Autodesk Inventor part; units mm, degrees
ref_plane "Work Plane1" through (0, 27, 0) normal (0, 1, 0) x (1, 0, 0)
ref_plane "YZ Plane" through (0, 0, 0) normal (1, 0, 0) x (0, 1, 0)
ref_plane "XZ Plane" through (0, 0, 0) normal (0, 1, 0) x (-1, 0, 0)
sketch "Sketch1" plane through (0, 0, 0) normal (0, 1, 0) x (-1, 0, 0)
  circle A0 centre (0, 0) radius 9.5
  circle A1 centre (0, 0) radius 13
  dimension "d0" = 19
  dimension "d3" = 26
extrude "Extrusion1" add sketch "Sketch1" against normal blind 6.5 contours A0
extrude "Extrusion2" add sketch "Sketch1" along normal blind 2 contours A0 | A1
sketch "Sketch2" plane through (0, 2, 0) normal (0, 1, 0) x (1, 0, 0)
  circle A0 centre (0, 0) radius 13
  circle A1 centre (0, 0) radius 10
  dimension "d6" = 20
ref_plane "Work Plane1" through (0, 27, 0) normal (0, 1, 0) x (1, 0, 0)
sketch "Sketch3" plane through (0, 27, 0) normal (0, 1, 0) x (1, 0, 0)
  circle A0 centre (0, 0) radius 2.5
  dimension "d8" = 5
loft "Loft1" add profiles "Sketch3", "Sketch2" contours all / A1
shell "Shell1" thickness 0.8 removed faces 2 at (1.2612, 27, 0.6619) at (-2.3703, -6.5, -2.0999)
properties part number "Microsuction"
For this review, take the finished solid that the model builds, in its own axes (mm). A direction names the side the tool comes from. Coordinates: 2 decimals unless noted, no trailing zeros. Write each loop counter-clockwise with the first axis right and the second up, starting at its lowest first coordinate (ties: lowest second). Pieces come first, ordered by that corner, then holes. Notation, with made-up numbers: (63, -35.75) - (88, -35.75) arc R11 cw to (88, -25.75) - close; hole circle Ø11 at (61.5, 19). An arc over 180 degrees is marked (long way). Put each result on its own line as item: value.
1. Mouldability with a two-part tool opening along Y and no side actions: class faces 6 (the cylindrical face through (10.316, 0.986, 7.91)), 7 (the flat face through (-8, 0.8, -5)), 8 (the conical face through (-4.34, 17.1, -3.33)) as released by +Y, released by -Y, zero draft, split by the parting line, or undercut.
Values found:
face 6: zero draft
face 7: undercut
face 8: released by +Y
2. Wall thickness on probe 1 along Z at (x, y) = (0, -2.5); probe 2 along Y at (x, z) = (-1.25, 10.75); probe 3 along X at (y, z) = (18.5, -2.25): over which ranges is each line inside the solid? List them lowest first.
Values found:
probe 1: -9.5 to -8.7, 8.7 to 9.5
probe 2: 0 to 0.8, 1.2 to 2
probe 3: -4.52 to -3.56, 3.56 to 4.52
3. Add section B-B, the plane y = 17. Give the boundary of the cut face in (x, z), then the cut area to 3 significant figures.
Values found:
outline: circle Ø11 at (0, 0); hole circle Ø9.33 at (0, 0)
area: 26.7 mm²
4. For pin 1 (13 mm diameter, centred on x = 4, z = -2, fed in from +Y); pin 2 (4 mm diameter, centred on x = -7, y = 6, fed in from +Z); pin 3 (12 mm diameter, centred on x = 3, y = 13, fed in from +Z); pin 4 (1.5 mm diameter, centred on x = -3.5, y = 8, fed in from -Z), all flat-tipped, find the tip position at first contact; note any pin that passes through.
Values found:
pin 1: y = 27
pin 2: z = 7.42
pin 3: z = 8.34
pin 4: z = -7.82
5. Add section A-A, the plane x = 0. Give the boundary of the cut face in (y, z), then the cut area to 3 significant figures.
Values found:
outline: (-6.5, -9.5) - (0, -9.5) - (0, -13) - (2, -13) - (2, -10) - (27, -2.5) - (27, -1.66) - (1.2, -9.4) - (1.2, -12.2) - (0.8, -12.2) - (0.8, -8.7) - (-6.5, -8.7) - close; (-6.5, 8.7) - (0.8, 8.7) - (0.8, 12.2) - (1.2, 12.2) - (1.2, 9.4) - (27, 1.66) - (27, 2.5) - (2, 10) - (2, 13) - (0, 13) - (0, 9.5) - (-6.5, 9.5) - close
area: 65.6 mm²
6. Machinability: for faces 1 (the flat face through (-7, 2, -8)), 2 (the flat face through (-4, -6.5, -8)), 3 (the flat face through (2, 27, 1)), 4 (the cylindrical face through (-4.38, -3.2, -8.43)), 5 (the flat face through (-6.3, 1.2, -7.2)), which of the approach directions +Z, -Z, +X, -X, +Y, -Y give a long, thin tool a straight path to every point of the face, cutting with its end or side? Answer none if there is none.
Values found:
face 1: +Y
face 2: +Z, -Z, +X, -X, -Y
face 3: +Z, -Z, +X, -X, +Y
face 4: -Y
face 5: none
7. Add section C-C, the plane y = 23. Give the boundary of the cut face in (x, z), then the cut area to 3 significant figures.
Values found:
outline: circle Ø7.4 at (0, 0); hole circle Ø5.73 at (0, 0)
area: 17.2 mm²
